from build123d import *

# Parameters (mm, degrees)
F0_W     = 42
F0_H     = 12.5
F1_DEPTH = 26
F2_R     = 3
F4_DEPTH = 24
F5_SIZE  = 1


with BuildPart() as f1:
    # F0 (on Top) → F1 (new body)
    with BuildSketch(Plane.XY):
        Rectangle(F0_W, F0_H)
    extrude(amount=F1_DEPTH)

    # F2
    f2_edges = [f1.edges().sort_by_distance(p)[0] for p in [
        (-21, 6.25, 13),
        (-21, -6.25, 13),
        (21, 6.25, 13),
        (21, -6.25, 13),
    ]]
    fillet(f2_edges, radius=F2_R)

    # F3 (on face) → F4 (cut)
    with BuildSketch(Plane.XY.offset(26)):
        with BuildLine():
            Line((18, 5.25), (-18, 5.25))
            ThreePointArc((-18, 5.25), (-19.4142135624, 4.6642135624), (-20, 3.25))
            Line((-20, 3.25), (-20, -3.25))
            ThreePointArc((-20, -3.25), (-19.4142135624, -4.6642135624), (-18, -5.25))
            Line((-18, -5.25), (18, -5.25))
            ThreePointArc((18, -5.25), (19.4142135624, -4.6642135624), (20, -3.25))
            Line((20, -3.25), (20, 3.25))
            ThreePointArc((20, 3.25), (19.4142135624, 4.6642135624), (18, 5.25))
        make_face()
    extrude(amount=-F4_DEPTH, mode=Mode.SUBTRACT)

    # F5
    f5_edges = [f1.edges().sort_by_distance(p)[0] for p in [
        (0, 6.25, 0),
        (20.12132, 5.37132, 0),
        (21, 0, 0),
        (20.12132, -5.37132, 0),
        (0, -6.25, 0),
        (-20.12132, -5.37132, 0),
        (-21, 0, 0),
        (-20.12132, 5.37132, 0),
    ]]
    chamfer(f5_edges, length=F5_SIZE)


solid = f1.part
Input: part model. Units: mm. Frame: model coordinates. A direction names the side the tool comes from. Give positions to 0.01 mm unless a question says otherwise; leave off trailing zeros. Write each loop counter-clockwise with the first axis right and the second up, starting at its lowest first coordinate (ties: lowest second). Pieces come first, ordered by that corner, then holes.
Q1. Pull-direction query (X, two-part tool) for faces 3 (the face through (19.71, -4.93, 0.4)), 4 (the face through (-20, 0, 14)), 5 (the face through (-19.71, 4.93, 0.4)), 6 (the face through (-19.4, 4.68, 14.17)); classes: pulls with the +X half, pulls with the -X half, needs draft (parallel to the pull), parting line crosses it, or undercut.
Q2. Section B-B, the plane y = 0.25. Output: boundary loops of the cut face in (x, z), plus the area to 3 significant figures.
Q3. Section A-A, the plane z = 21.5. Output: boundary loops of the cut face in (x, y), plus the area to 3 significant figures.
Q4. Material intervals for probe 1 along X at (y, z) = (-2, 22.25); probe 2 along Y at (x, z) = (15.5, 13.25); probe 3 along Z at (x, y) = (9, 1.25), sorted ascending.
Q5. Section C-C, the plane x = -9.5. Output: boundary loops of the cut face in (y, z).
Q6. First-contact query: P1, Ø3, axis at x = -3.5, y = 0.5, coming from the +Z side. Flat tip, straight axial feed; report the tip coordinate or a pass-through.
Q7. Set-up query: faces 1 (the face through (0, -5.25, 14)), 2 (the face through (19.68, 4.96, 0.4)). Return all of +Z, -Z, +X, -X, +Y, -Y with unobstructed straight access to the full face (end or side cutting, diameter ignored); none if empty.
Filled in:
1. face 3: pulls with the +X half
1. face 4: undercut
1. face 5: pulls with the -X half
1. face 6: undercut
2. outline: (-21, 1) - (-20, 0) - (20, 0) - (21, 1) - (21, 26) - (20, 26) - (20, 2) - (-20, 2) - (-20, 26) - (-21, 26) - close
2. area: 131 mm2
3. outline: (-21, -3.25) arc R3 ccw to (-18, -6.25) - (18, -6.25) arc R3 ccw to (21, -3.25) - (21, 3.25) arc R3 ccw to (18, 6.25) - (-18, 6.25) arc R3 ccw to (-21, 3.25) - close; hole (-20, -3.25) arc R2 ccw to (-18, -5.25) - (18, -5.25) arc R2 ccw to (20, -3.25) - (20, 3.25) arc R2 ccw to (18, 5.25) - (-18, 5.25) arc R2 ccw to (-20, 3.25) - close
3. area: 101 mm2
4. probe 1: x = -21 to -20, 20 to 21
4. probe 2: y = -6.25 to -5.25, 5.25 to 6.25
4. probe 3: z = 0 to 2
5. outline: (-6.25, 1) - (-5.25, 0) - (5.25, 0) - (6.25, 1) - (6.25, 26) - (5.25, 26) - (5.25, 2) - (-5.25, 2) - (-5.25, 26) - (-6.25, 26) - close
6. P1: stops at z = 2
7. face 1: +Z
7. face 2: -Z, +X, +Y
